Geometry: final body of the model. Coordinates: model frame, mm. Face numbers are marked on the shaded views. A direction names the side the tool comes from. Coordinates: 2 decimals unless noted, no trailing zeros. Loops run counter-clockwise (first coordinate to the right, second up) from the corner with the lowest first, then second, coordinate; pieces in that order, holes last. Notation, with made-up numbers: (48.25, -22) -> (97.25, -22) arc R17 cw to (97.25, -16) -> close; hole circle Ø3 at (56.5, 50.5). An arc over 180 degrees is marked (long way). One line per item, written item: value. Start each with the question number.
Autodesk Inventor part; units mm, degrees
ref_plane "YZ Plane" through (0, 0, 0) normal (1, 0, 0) x (0, 1, 0)
ref_plane "XZ Plane" through (0, 0, 0) normal (0, 1, 0) x (-1, 0, 0)
ref_plane "XY Plane" through (0, 0, 0) normal (0, 0, 1) x (1, 0, 0)
sketch "Sketch1" plane through (0, 0, 0) normal (0, 0, 1) x (1, 0, 0)
  circle A0 centre (0, -228.6) radius 228.6 construction
  line L0 (0, 0) -> (0, 15) construction
  line L1 (0, 15) -> (-3, 15) construction
  line L2 (0, 0) -> (-100, 0) construction
  line L3 (0, 0) -> (0, -85) construction
  line L4 (0, 15) -> (0, 30) construction
  line L5 (0, -85) -> (-177.8679, -85) construction
  line L6 (-177.8679, -85) -> (-196.774, -85) construction
  circle A1 centre (0, -228.6) radius 243.6 construction
  circle A2 centre (0, -228.6) radius 258.6 construction
  arc A3 (0, 30) -> (-215.0651, -85) centre (0, -228.6) ccw
  line L7 (-30, -1.9771) -> (0, 30)
  line L8 (-118.8814, -33.3433) -> (-139.0909, -28.6133)
  line L9 (-196.774, -85) -> (-215.0651, -85) construction
  line L10 (-215.0651, -85) -> (-196.774, -85)
  arc A4 (-139.0909, -28.6133) -> (-196.774, -85) centre (0, -228.6) ccw
  circle A5 centre (0, -228.6) radius 233.6 construction
  circle A6 centre (0, -228.6) radius 253.6 construction
  line L11 (-119.7215, -28.0115) -> (-146.6573, -21.7073)
  line L12 (-32.4328, 2.7376) -> (-11.8047, 24.7251)
  arc A7 (-32.4328, 2.7376) -> (-119.7215, -28.0115) centre (0, -228.6) ccw
  arc A8 (-11.8047, 24.7251) -> (-146.6573, -21.7073) centre (0, -228.6) ccw
  line L13 (-118.8814, -33.3433) -> (0, -228.6) construction
  line L14 (-30, -1.9771) -> (0, -228.6) construction
  line L15 (-118.8814, -33.3433) -> (-103.2801, -58.9675)
  line L16 (-30, -1.9771) -> (-26.063, -31.7176)
  line L17 (-103.2801, -58.9675) -> (-26.063, -31.7176)
  line L18 (-114.6107, -30.7431) -> (-101.1189, -52.9026)
  line L19 (-101.1189, -52.9026) -> (-31.5521, -28.3525)
  line L20 (-31.5521, -28.3525) -> (-34.9568, -2.6332)
  arc A9 (-34.9568, -2.6332) -> (-114.6107, -30.7431) centre (0, -228.6) ccw
  dimension "d2" = 457.2
  dimension "d3" = 228.6
  dimension "d6" = 3
  dimension "d7" = 100
  dimension "d9" = 85
  dimension "d13" = 15
  dimension "d14" = 15
  dimension "d18" = 30
  dimension "d21" = 120
  dimension "d22" = 20.2095
  dimension "d23" = 467.2
  dimension "d24" = 507.2
  dimension "d25" = 5
  dimension "d26" = 5
  dimension "d27" = 30
  dimension "d28" = 30
  dimension "d29" = 5
  dimension "d30" = 228.6547
extrude "Extrusion1" add sketch "Sketch1" along normal blind 14
fillet "Fillet1" radius 5 14 edges at (-30, -1.9771, 7) (-118.8814, -33.3433, 7) (-139.0909, -28.6133, 7) (-11.8047, 24.7251, 7) (-146.6573, -21.7073, 7) (0, 30, 7) (-32.4328, 2.7376, 7) (-101.1189, -52.9026, 7) (-31.5521, -28.3525, 7) (-119.7215, -28.0115, 7) (-196.774, -85, 7) (-215.0651, -85, 7) (-26.063, -31.7176, 7) (-103.2801, -58.9675, 7)
sketch "Sketch2" plane through (-26.5953, -27.6963, 14) normal (0.9914, 0.1312, 0) x (0, 0, -1)
  line L0 (5, 4.0564) -> (9, 4.0564)
  line L1 (9, 4.0564) -> (9, 12.0564)
  line L2 (9, 12.0564) -> (5, 12.0564)
  line L3 (5, 12.0564) -> (5, 4.0564)
  line L4 (14, 0) -> (14, 23.5741)
  line L5 (0, 0) -> (0, 23.5741)
  line L6 (5, 12.0564) -> (9, 12.0564)
  line L7 (5, 4.0564) -> (9, 4.0564)
  line L8 (0, 4.0564) -> (14, 4.0564)
  point P0 (14, 23.9666)
  dimension "d34" = 5
  dimension "d35" = 5
  dimension "d46" = 8
extrude "Extrusion2" cut sketch "Sketch2" against normal blind 5
sketch "Sketch3" plane through (-105.3896, -55.5028, 0) normal (-0.8541, -0.52, 0) x (0, 0, 1)
  line L0 (9, 14.0564) -> (9, 4.0564)
  line L1 (9, 4.0564) -> (5, 4.0564)
  line L2 (0, 4.0564) -> (14, 4.0564)
  line L3 (5, 14.0564) -> (9, 14.0564)
  line L4 (14, 4.0564) -> (14, 25.9436)
  line L5 (5, 4.0564) -> (5, 14.0564)
  line L6 (0, 25.9436) -> (0, 4.0564)
  point P0 (0, -7.3997)
  dimension "d38" = 5
  dimension "d39" = 5
  dimension "d40" = 10
  dimension "d41" = 10
  dimension "d42" = 90
extrude "Extrusion3" cut sketch "Sketch3" against normal blind 5
properties part number "Bumper" material "ABS Plastic"
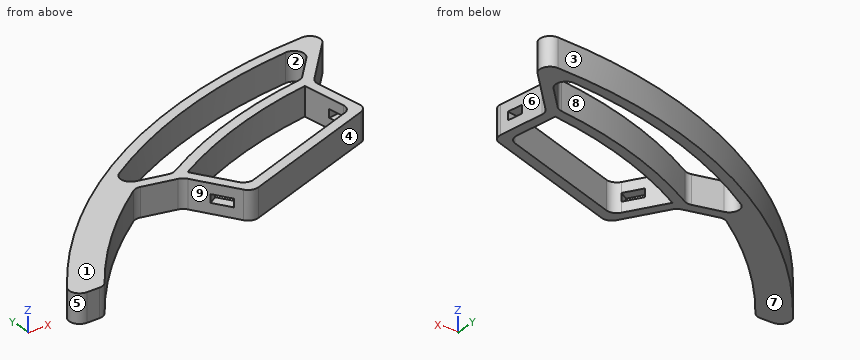
1. Line query: L1, parallel to Y at x = -63.5, z = 12.75; L2, parallel to Y at x = -72, z = 1.75; L3, parallel to Y at x = -124.5, z = 8.25. Output: solid intervals per line, ascending. Write a range as [from, to].
2. Draft query along X for the marked faces 1, 2, 3 and 4. Return one class per face: released by +X, released by -X, zero draft, split by the parting line, or undercut.
3. Section B-B on y = 7.5. Return the cut outline in (x, z), plus the area to 3 significant figures.
4. Pin query (flat end, axial travel): pin 1 Ø1 at (y, z) = (-7, 12) entering from +X; pin 2 Ø5 at (y, z) = (13.5, 1.5) entering from +X; pin 3 Ø1.5 at (x, z) = (-115, 6) entering from -Y. Return the tip coordinate at first contact, or that it passes through.
5. Set-up query: the marked faces 5, 6, 7, 8 and 9. Return all of +Z, -Z, +X, -X, +Y, -Y with unobstructed straight access to the full face (end or side cutting, diameter ignored); none if empty.
6. Section D-D on y = -11.5. Return the cut outline in (x, z).
7. Section C-C on z = 2.75. Count the separate pieces of the cut face and the enclosed holes in it, plus the area to 3 significant figures.
8. Section A-A on x = -127. Return the cut outline in (y, z).
Checks:
1. L1: [-44.93, -39.63], [-8.94, -3.8], [16.92, 22.08]
1. L2: [-47.93, -42.63], [-11.58, -6.37], [14.56, 19.77]
1. L3: [-32.03, -26.89], [-7.66, -1.94]
2. face 1: zero draft
2. face 2: undercut
2. face 3: released by -X
2. face 4: released by +X
3. outline: (-105.5, 0) -> (-92.57, 0) -> (-92.57, 14) -> (-105.5, 14) -> close; (-27.96, 0) -> (-21.11, 0) -> (-21.11, 14) -> (-27.96, 14) -> close
3. area: 277 mm²
4. pin 1: x = -29.27
4. pin 2: x = -13.13
4. pin 3: y = -40.95
5. face 5: +Z, -Z, -X
5. face 6: +Z, -Z, +X
5. face 7: -Z, +X, -X, +Y, -Y
5. face 8: +Z, -Z
5. face 9: +Z, -Z, -Y
6. outline: (-140.5, 0) -> (-131.07, 0) -> (-131.07, 14) -> (-140.5, 14) -> close; (-86.24, 0) -> (-71.77, 0) -> (-71.77, 14) -> (-86.24, 14) -> close; (-33.78, 0) -> (-28.74, 0) -> (-28.74, 14) -> (-33.78, 14) -> close
7. separate pieces: 1
7. enclosed holes: 2
7. area: 3,530 mm²
8. outline: (-31.44, 0) -> (-26.31, 0) -> (-26.31, 14) -> (-31.44, 14) -> close; (-9.09, 0) -> (-3.33, 0) -> (-3.33, 14) -> (-9.09, 14) -> close
